```python
from build123d import *

# Parameters (mm, degrees)
PIPE_1_PROFILE_R   = 11
EXTRUDE_SKETCH_1_R = 17
EXTRUDE_1_DEPTH    = 4
EXTRUDE_SKETCH_2_R = 17
EXTRUDE_2_DEPTH    = 4


with BuildPart() as part:
    # Pipe 1: sweep along a curve in space
    with BuildLine() as pipe_1_path:
        Line((-60, 0, 0), (-60, 0, 33))
        ThreePointArc((-60, 0, 33), (-53.556349186, 0, 48.556349186), (-38, 0, 55))
        Line((-38, 0, 55), (38, 0, 55))
        ThreePointArc((38, 0, 55), (53.556349186, 0, 48.556349186), (60, 0, 33))
        Line((60, 0, 33), (60, 0, 0))
    # Pipe 1 profile (on start of the path) → Pipe 1 (sweep)
    with BuildSketch(Plane(origin=(-60, 0, 0), x_dir=(1, 0, 0), z_dir=(0, 0, 1))):
        Circle(PIPE_1_PROFILE_R)
    sweep(path=pipe_1_path.line)


with BuildPart() as body_2:
    # Extrude sketch 1 → Extrude 1 (new body)
    with BuildSketch(Plane.XY):
        with Locations((-60, 0)):
            Circle(EXTRUDE_SKETCH_1_R)
    extrude(amount=EXTRUDE_1_DEPTH)


with BuildPart() as body_3:
    # Extrude sketch 2 → Extrude 2 (new body)
    with BuildSketch(Plane.XY):
        with Locations((60, 0)):
            Circle(EXTRUDE_SKETCH_2_R)
    extrude(amount=EXTRUDE_2_DEPTH)


with BuildPart() as body_2_1:
    add(body_2.part)

    # Combine (weld / assembly of features): union body 3, part
    add(body_3.part)
    add(part.part)


solid = body_2_1.part
```
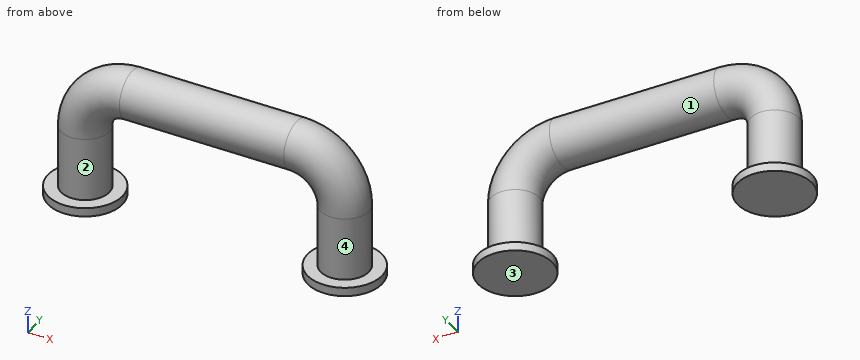
CAD build for the part. Positions are in the model's coordinates, mm. Face numbers are marked on the shaded views. Give positions to 0.01 mm unless a question says otherwise; leave off trailing zeros. Order: outer loops, then holes, each group sorted by start corner. A loop starts at its lowest first (then second) coordinate and runs counter-clockwise, first axis right, second up.
(1) Drill centre lines: L1, parallel to Z at x = -47.5, y = -2; L2, parallel to Z at x = 50.5, y = -14; L3, parallel to X at y = 4, z = 5. Where is each one in solid material? Low to high.
(2) Mould opens along Z. For the marked faces 1, 2, 3 and 4 say: released by +Z, released by -Z, zero draft, split by the parting line, or undercut.
(3) Saw through at B-B, the plane y = 14. Give the cut face in (x, z).
(4) Flat gauge pins, fed straight in: pin 1 (12 mm diameter, centred on x = 31, y = 4.5, fed in from -Z); pin 2 (6 mm diameter, centred on y = 0.5, z = 24.5, fed in from -X); pin 3 (2 mm diameter, centred on x = -28, y = 9.5, fed in from -Z). Where does each tip first touch, or does it go through?
(5) Saw through at C-C, the plane x = -13.5. Give the cut face in (y, z).
(6) Saw through at A-A, the plane y = 0. Give the cut face in (x, z), then the cut area to 3 significant figures.
Results found:
1. L1: z = 0 to 4, 38.9 to 64.41
1. L2: z = 0 to 4
1. L3: x = -70.25 to -49.75, 49.75 to 70.25
2. face 1: split by the parting line
2. face 2: undercut
2. face 3: released by -Z
2. face 4: undercut
3. outline: (-69.64, 0) - (-50.36, 0) - (-50.36, 4) - (-69.64, 4) - close; (50.36, 0) - (69.64, 0) - (69.64, 4) - (50.36, 4) - close
4. pin 1: stops at z = 44
4. pin 2: stops at x = -71
4. pin 3: stops at z = 48.02
5. outline: circle Ø22 at (0, 55)
6. outline: (-77, 0) - (-43, 0) - (-43, 4) - (-49, 4) - (-49, 33) arc R11 cw to (-38, 44) - (38, 44) arc R11 cw to (49, 33) - (49, 4) - (43, 4) - (43, 0) - (77, 0) - (77, 4) - (71, 4) - (71, 33) arc R33 ccw to (38, 66) - (-38, 66) arc R33 ccw to (-71, 33) - (-71, 4) - (-77, 4) - close
6. area: 4,740 mm2
